Could you check a few things on this model? Use its own coordinates, in mm. A direction names the side the tool comes from. Give positions to 0.01 mm unless a question says otherwise; leave off trailing zeros. Loops run counter-clockwise (first coordinate to the right, second up) from the corner with the lowest first, then second, coordinate; pieces in that order, holes last. Notation, with made-up numbers: (36, 24.5) -> (68, 24.5) arc R34 ccw to (68, 60.5) -> close; hole circle Ø2 at (-25.75, 20). An arc over 180 degrees is marked (long way). Put each result on its own line as item: value.
```python
from build123d import *

# Parameters (mm, degrees)
SKETCH_1_R                   = 6
SKETCH_1_R_2                 = 1.5
SKETCH_1_W                   = 25
SKETCH_1_H                   = 18
EXTRUDE_1_DEPTH              = 8
HOLE_WIZARD_M3_1_D           = 2.5
HOLE_WIZARD_M3_1_DEPTH       = 6.748924226
HOLE_WIZARD_M3_1_CSINK_D     = 3.05
HOLE_WIZARD_M3_1_CSINK_ANGLE = 45
HOLE_WIZARD_M3_1_TIP         = 0.751075774
HOLE_WIZARD_M3_2_D           = 2.5
HOLE_WIZARD_M3_2_CSINK_D     = 3.05
HOLE_WIZARD_M3_2_CSINK_ANGLE = 45


with BuildPart() as part:
    # 草圖1 → 填料-伸長1 (new body)
    with BuildSketch(Plane.XY):
        with BuildLine():
            Line((-52.401923789, -30.5), (-30.462613559, 7.5))
            ThreePointArc((-30.462613559, 7.5), (-28.632486541, 9.330127019), (-26.132486541, 10))
            Line((-26.132486541, 10), (0, 10))
            Line((0, 10), (20, 10))
            Line((20, 10), (20, -35))
            Line((20, -35), (0, -35))
            Line((0, -35), (-49.803847577, -35))
            ThreePointArc((-49.803847577, -35), (-52.401923789, -33.5), (-52.401923789, -30.5))
        make_face()
        Circle(SKETCH_1_R, mode=Mode.SUBTRACT)
        with Locations((-32, -5)):
            Circle(SKETCH_1_R_2, mode=Mode.SUBTRACT)
        with Locations((-32, -15)):
            Circle(SKETCH_1_R_2, mode=Mode.SUBTRACT)
        with Locations((-32, -25)):
            Circle(SKETCH_1_R_2, mode=Mode.SUBTRACT)
        with Locations((0, -20.5)):
            Rectangle(SKETCH_1_W, SKETCH_1_H, mode=Mode.SUBTRACT)
    extrude(amount=EXTRUDE_1_DEPTH)

    # M3 螺紋孔1
    with Locations(Plane(origin=(-10, -35, 4), x_dir=(0, 0, -1), z_dir=(0, -1, 0))):
        with Locations((0, 0), (0, 15), (0, -15)):
            CounterSinkHole(HOLE_WIZARD_M3_1_D / 2, HOLE_WIZARD_M3_1_CSINK_D / 2, depth=HOLE_WIZARD_M3_1_DEPTH, counter_sink_angle=HOLE_WIZARD_M3_1_CSINK_ANGLE)
            with Locations((0, 0, -(HOLE_WIZARD_M3_1_DEPTH + HOLE_WIZARD_M3_1_TIP / 2))):  # 118° drill point
                Cone(0, HOLE_WIZARD_M3_1_D / 2, HOLE_WIZARD_M3_1_TIP, mode=Mode.SUBTRACT)

    # M3 螺紋孔2 (through all)
    with Locations(Plane(origin=(15, 0, 0), x_dir=(-1, 0, 0), z_dir=(0, 0, -1))):
        with Locations((0, 0), (30, 0)):
            CounterSinkHole(HOLE_WIZARD_M3_2_D / 2, HOLE_WIZARD_M3_2_CSINK_D / 2, counter_sink_angle=HOLE_WIZARD_M3_2_CSINK_ANGLE)


solid = part.part
```
1. If we section it at C-C (x = 10): List the corners of the cut face in (y, z) for me, then the cut area to 3 significant figures.
Recorded:
outline: (-35, 0) -> (-29.5, 0) -> (-29.5, 8) -> (-35, 8) -> close; (-11.5, 0) -> (10, 0) -> (10, 8) -> (-11.5, 8) -> close
area: 216 mm^2
2. I'm going to push flat-ended pins straight in: pin 1 (2.5 mm diameter, centred on x = -32, y = -15, fed in from -Z); pin 2 (12 mm diameter, centred on x = -40, y = 2.5, fed in from +Z). Where does each tip first touch, or does it pass through?
Recorded:
pin 1: passes through
pin 2: stops at z = 8
3. If we section it at D-D (y = -15): List the corners of the cut face in (x, z) for me, then the cut area to 3 significant figures.
Recorded:
outline: (-43.45, 0) -> (-33.5, 0) -> (-33.5, 8) -> (-43.45, 8) -> close; (-30.5, 0) -> (-12.5, 0) -> (-12.5, 8) -> (-30.5, 8) -> close; (12.5, 0) -> (20, 0) -> (20, 8) -> (12.5, 8) -> close
area: 284 mm^2
4. If we section it at B-B (z = 1.5): List the corners of the cut face in (x, y) for me, then the cut area to 3 significant figures.
Recorded:
outline: (-52.4, -30.5) arc R3 ccw to (-49.8, -35) -> (20, -35) -> (20, 10) -> (-26.13, 10) arc R5 ccw to (-30.46, 7.5) -> close; hole circle Ø3 at (-32, -25); hole circle Ø3 at (-32, -15); hole circle Ø3 at (-32, -5); hole circle Ø2.5 at (-15, 0); hole (-12.5, -29.5) -> (12.5, -29.5) -> (12.5, -11.5) -> (-12.5, -11.5) -> close; hole circle Ø12 at (0, 0); hole circle Ø2.5 at (15, 0)
area: 2,190 mm^2
5. If we section it at A-A (x = -10): List the corners of the cut face in (y, z) for me (3 decimals), then the cut area to 3 significant figures.
Recorded:
outline: (-35, 0) -> (-29.5, 0) -> (-29.5, 2.75) -> (-34.336, 2.75) -> (-35, 2.475) -> close; (-35, 5.525) -> (-34.336, 5.25) -> (-29.5, 5.25) -> (-29.5, 8) -> (-35, 8) -> close; (-11.5, 0) -> (10, 0) -> (10, 8) -> (-11.5, 8) -> close
area: 202 mm^2
6. Thinking about a two-plate mould opening in Z: for faces 1 (the face through (-6, 0, 4)), 2 (the face through (-16, -12, 0)), 3 (the face through (-24.785, -27.63, 4.028)), which applies, pulls with the +Z half, pulls with the -Z half, needs draft (parallel to the pull), parting line crosses it, or undercut?
Recorded:
face 1: needs draft
face 2: pulls with the -Z half
face 3: undercut
7. I need wall thicknesses on line 1 (X direction, y = -30.5, z = 4); line 2 (Z direction, x = -25, y = -32); line 3 (X direction, y = -14, z = 3). Which ranges of each line are inside material? Lowest first, please.
Recorded:
line 1: x = -52.4 to -26.25, -23.75 to -11.25, -8.75 to 3.75, 6.25 to 20
line 2: z = 0 to 2.75, 5.25 to 8
line 3: x = -42.88 to -33.12, -30.88 to -12.5, 12.5 to 20
8. For faces 4 (the face through (-26.22, -31.25, 3.73)), 5 (the face through (12.5, -21, 4)), 6 (the face through (-3, 10, 4)), which set-ups out of +Z, -Z, +X, -X, +Y, -Y let a thin tool reach every point of the face, with its end or its side?
Recorded:
face 4: -Y
face 5: +Z, -Z
face 6: +Z, -Z, +X, -X, +Y
